Source: CAD feature listing. Evaluate the final solid. Frame: model axes, mm. Face numbers are marked on the shaded views. A direction names the side the tool comes from. Give positions to 0.01 mm unless a question says otherwise; leave off trailing zeros. Write each loop counter-clockwise with the first axis right and the second up, starting at its lowest first coordinate (ties: lowest second). Pieces come first, ordered by that corner, then holes.
```python
from build123d import *

# Parameters (mm, degrees)
F0_W      = 94
F0_H      = 45
F1_DEPTH  = 2
F2_W      = 2
F2_H      = 45
F3_DEPTH  = 16
F4_W      = 94
F4_H      = 18
F5_DEPTH  = 2
F6_W      = 2
F6_H      = 6
F7_DEPTH  = 11
F8_R      = 1.25
F8_R_2    = 1.5
F9_DEPTH  = 25
F10_R     = 2
F12_W     = 19.2678107619
F12_H     = 14.8564111814
F12_W_2   = 16.8835728168
F12_H_2   = 15.2771589719
F13_DEPTH = 25
F14_R     = 1.5
F15_DEPTH = 100
F16_R     = 1.5
F17_DEPTH = 100
F18_SIZE  = 1.87
F19_W     = 84
F19_H     = 28
F20_DEPTH = 25


with BuildPart() as f1:
    # F0 (on Front) → F1 (new body)
    with BuildSketch(Plane.XZ):
        Rectangle(F0_W, F0_H)
    extrude(amount=F1_DEPTH)

    # F2 (on face) → F3 (join)
    with BuildSketch(Plane(origin=(0, 0, 0), x_dir=(-1, 0, 0), z_dir=(0, 1, 0))):
        with Locations((-46, 0)):
            Rectangle(F2_W, F2_H)
        with Locations((46, 0)):
            Rectangle(F2_W, F2_H)
    extrude(amount=F3_DEPTH)

    # F4 (on face) → F5 (join)
    with BuildSketch(Plane.XY.offset(22.5)):
        with Locations((0, 7)):
            Rectangle(F4_W, F4_H)
    extrude(amount=-F5_DEPTH)

    # F6 (on face) → F7 (join)
    with BuildSketch(Plane.YZ.offset(47)):
        with Locations((15, 16)):
            Rectangle(F6_W, F6_H)
        with Locations((15, -16)):
            Rectangle(F6_W, F6_H)
    extrude(amount=F7_DEPTH)

    # F8 (on face) → F9 (cut)
    with BuildSketch(Plane.XZ.offset(-14)):
        with Locations((53.5, 16)):
            Circle(F8_R)
        with Locations((53.5, -16)):
            Circle(F8_R_2)
    extrude(amount=-F9_DEPTH, mode=Mode.SUBTRACT)

    # F10
    f10_edges = [f1.edges().sort_by_distance(p)[0] for p in [
        (58, 15, -19),
        (58, 15, -13),
        (58, 15, 19),
        (58, 15, 13),
        (47, 14, -16),
        (47, 14, 16),
    ]]
    fillet(f10_edges, radius=F10_R)

    # F11: F1 across plane


with BuildPart() as f1_1:
    add(f1.part)
    add(f1.part.mirror(Plane.YZ))

    # F12 (on face) → F13 (cut)
    with BuildSketch(Plane.XZ.offset(2)):
        with Locations((56.633905381, -15.0717944093)):
            Rectangle(F12_W, F12_H)
        with Locations((-55.4417864084, -14.8614205141)):
            Rectangle(F12_W_2, F12_H_2)
    extrude(amount=-F13_DEPTH, mode=Mode.SUBTRACT)

    # F14 (on face) → F15 (cut)
    with BuildSketch(Plane(origin=(-47, 0, 0), x_dir=(0, -1, 0), z_dir=(-1, 0, 0))):
        with Locations((-9.5, -16)):
            Circle(F14_R)
    extrude(amount=-F15_DEPTH, mode=Mode.SUBTRACT)

    # F16 (on face) → F17 (cut)
    with BuildSketch(Plane(origin=(-47, 0, 0), x_dir=(0, -1, 0), z_dir=(-1, 0, 0))):
        with Locations((-9.5, 8)):
            Circle(F16_R)
    extrude(amount=-F17_DEPTH, mode=Mode.SUBTRACT)

    # F18
    f18_edges = [f1_1.edges().sort_by_distance(p)[0] for p in [
        (45, 11, 8),
        (45, 11, -16),
        (-45, 11, 8),
        (-45, 11, -16),
    ]]
    chamfer(f18_edges, length=F18_SIZE)

    # F19 (on face) → F20 (cut)
    with BuildSketch(Plane.XZ.offset(2)):
        with Locations((0, -22.5)):
            Rectangle(F19_W, F19_H)
    extrude(amount=-F20_DEPTH, mode=Mode.SUBTRACT)


solid = f1_1.part
```
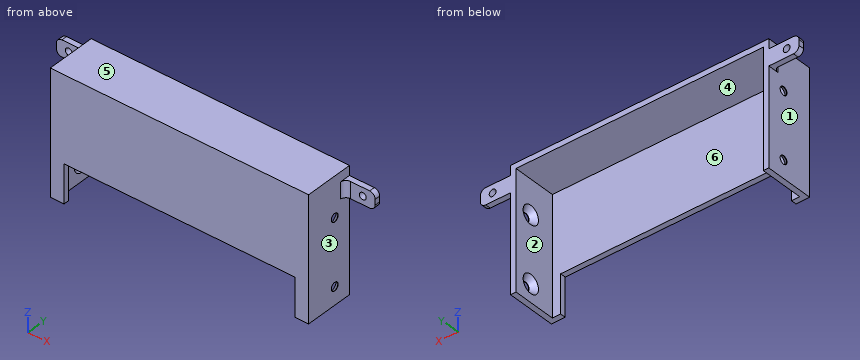
1. Section query B-B (x = 53.5). Return loops of the section in (y, z).
2. Pin query (flat end, axial travel): P1, Ø1, axis at y = -1, z = -18, coming from the -X side; P2, Ø1.5, axis at x = 19.5, z = -1, coming from the +Y side; P3, Ø1.8, axis at x = 52.5, z = 15.5, coming from the -Y side. Return the tip coordinate at first contact, or that it passes through.
3. Section query C-C (z = -16). Return loops of the section in (x, y).
4. Pull-direction query (X, two-part tool) for the marked faces 1, 2, 3 and 4; classes: pulls with the +X half, pulls with the -X half, needs draft (parallel to the pull), parting line crosses it, or undercut.
5. Access query for the marked faces 5 and 6. Directions: +Z, -Z, +X, -X, +Y, -Y. A direction counts if a zero-diameter tool reaches every point of the face in a straight line with its end or side. Return the directions, or none.
6. Section query D-D (z = 8). Return loops of the section in (x, y), plus the area to 3 significant figures.
7. Section query A-A (y = 9.5). Give the number of separate pieces and of enclosed holes in the cut face, plus the area to 3 significant figures.
8. Line query: probe 1 along Z at (x, y) = (46.95, 9.5); probe 2 along X at (y, z) = (1.5, -14); probe 3 along Z at (x, y) = (1.5, 1). Output: solid intervals per line, ascending.
The answers:
1. outline: (14, 13) - (16, 13) - (16, 14.75) - (14, 14.75) - close; (14, 17.25) - (16, 17.25) - (16, 19) - (14, 19) - close
2. P1: stops at x = -47
2. P2: stops at y = 0
2. P3: stops at y = 14
3. outline: (-47, -2) - (-42, -2) - (-42, 0) - (-45, 0) - (-45, 6.13) - (-46.87, 8) - (-47, 8) - close; (-47, 11) - (-46.87, 11) - (-45, 12.87) - (-45, 16) - (-47, 16) - close; (42, -2) - (47, -2) - (47, 8) - (46.87, 8) - (45, 6.13) - (45, 0) - (42, 0) - close; (45, 12.87) - (46.87, 11) - (47, 11) - (47, 16) - (45, 16) - close
4. face 1: pulls with the -X half
4. face 2: undercut
4. face 3: pulls with the +X half
4. face 4: undercut
5. face 5: +Z, +X, -X, +Y, -Y
5. face 6: -Z, +Y
6. outline: (-47, -2) - (47, -2) - (47, 8) - (46.87, 8) - (45, 6.13) - (45, 0) - (-45, 0) - (-45, 6.13) - (-46.87, 8) - (-47, 8) - close; (-47, 11) - (-46.87, 11) - (-45, 12.87) - (-45, 16) - (-47, 16) - close; (45, 12.87) - (46.87, 11) - (47, 11) - (47, 16) - (45, 16) - close
6. area: 233 mm2
7. separate pieces: 5
7. enclosed holes: 0
7. area: 322 mm2
8. probe 1: z = -22.5 to -17.5, -14.5 to 6.5, 9.5 to 22.5
8. probe 2: x = -47 to -45, 45 to 47
8. probe 3: z = 20.5 to 22.5
